The model under review builds one solid part; all positions refer to its coordinate system, in mm. Round coordinates to 2 decimals unless told otherwise and drop trailing zeros. Answer in a Markdown table with one row per item. Add a question column.
```python
from build123d import *

# Parameters (mm, degrees)
F0_W     = 320
F0_H     = 320
F1_DEPTH = 25
F2_R     = 125
F3_DEPTH = 20
F4_R     = 10


with BuildPart() as f1:
    # F0 (on Top) → F1 (new body)
    with BuildSketch(Plane.XY):
        with Locations((6.127898, 10.826058)):
            Rectangle(F0_W, F0_H)
    extrude(amount=F1_DEPTH)


with BuildPart() as f3:
    # F2 (on face) → F3 (new body)
    with BuildSketch(Plane.XY.offset(25)):
        with Locations((357.512802, 15.676551)):
            Circle(F2_R)
    extrude(amount=F3_DEPTH)

    # F4
    f4_edges = [f3.edges().sort_by_distance(p)[0] for p in [
        (232.512802, 15.676551, 25),
    ]]
    fillet(f4_edges, radius=F4_R)


with BuildPart() as f3_1:
    # F5: moved
    add(f3.part.moved(Location((-342, 0, -16))))


with BuildPart() as f1_1:
    add(f1.part)

    # F6: cut F3
    add(f3_1.part, mode=Mode.SUBTRACT)


solid = f1_1.part
```
1. For L1, parallel to Z at x = 45, y = 65.5; L2, parallel to Y at x = -64, z = 19; L3, parallel to Y at x = -44, z = 20.25, list the stretches that pass through material, from the lowest coordinate up.
2. Insertion check: pin 1 Ø2 at (x, y) = (-3.5, 63) entering from +Z. The pin has a flat end and moves straight along its axis. Give the tip position at first contact, or say it passes through.
3. Mouldability with a two-part tool opening along X and no side actions: class faces 1 (the flat face through (14, 17, 9)), 2 (the flat face through (166.128, 9, 12)), 3 (the cylindrical face through (-0.76, 139.613, 21.958)), 4 (the flat face through (4, -149.174, 12)) as pulls with the +X half, pulls with the -X half, needs draft (parallel to the pull), parting line crosses it, or undercut.
Filled in:
| question | item | result |
|---|---|---|
| 1 | L1 | 0 to 9 |
| 1 | L2 | -149.17 to -80.77, 112.13 to 170.83 |
| 1 | L3 | -149.17 to -94.25, 125.6 to 170.83 |
| 2 | pin 1 | z = 9 |
| 3 | face 1 | undercut |
| 3 | face 2 | pulls with the +X half |
| 3 | face 3 | undercut |
| 3 | face 4 | needs draft |
